Autodesk Inventor part; units mm, degrees
ref_plane "YZ Plane" through (0, 0, 0) normal (1, 0, 0) x (0, 1, 0)
ref_plane "XZ Plane" through (0, 0, 0) normal (0, 1, 0) x (-1, 0, 0)
ref_plane "XY Plane" through (0, 0, 0) normal (0, 0, 1) x (1, 0, 0)
sketch "Sketch1" plane through (0, 0, 0) normal (0, 0, 1) x (1, 0, 0)
  line L0 (45, 15) -> (-5, 15)
  line L1 (-1, 8) -> (-1, 0)
  line L2 (1, 0) -> (1, 8)
  arc A0 (1, 8) -> (-1, 8) centre (0, 8) ccw
  arc A1 (17, 8) -> (15, 8) centre (16, 8) ccw
  line L3 (15, 8) -> (15, 0)
  line L4 (17, 0) -> (17, 8)
  line L5 (2.5, 0) -> (2.5, 0)
  line L6 (22.48, 0) -> (22.48, 0)
  line L7 (-5, 15) -> (-5, 0)
  line L8 (-5, 0) -> (-1, 0)
  line L9 (45, 0) -> (45, 15)
  line L10 (17, 0) -> (45, 0)
  line L11 (1, 0) -> (15, 0)
  point P0 (0, 0)
  point P1 (15, 0)
  dimension "d0" = 50
  dimension "d1" = 15
  dimension "d3" = 2
  dimension "d6" = 0
  dimension "d7" = 16
extrude "Extrusion2" add sketch "Sketch1" along normal blind 3.5
properties part number "C2"
Geometry check sheet. Reference: the model listing, model coordinates, mm. A direction names the side the tool comes from. Round coordinates to 2 decimals unless told otherwise and drop trailing zeros. Write each loop counter-clockwise with the first axis right and the second up, starting at its lowest first coordinate (ties: lowest second). Pieces come first, ordered by that corner, then holes. Notation, with made-up numbers: (14.5, 34) -> (56.5, 34) arc R9 cw to (56.5, 45) -> close; hole circle Ø10 at (25.25, -26). An arc over 180 degrees is marked (long way). One line per item, written item: value. Start each with the question number.
(1) Cross-section at B-B, the plane z = 1.95. Record the cut outline in (x, y), and give its area (3 significant figures).
(2) Draft check along X on faces 3 (the flat face through (-3, 0, 2)), 4 (the cylindrical face through (0, 9, 2)), 5 (the flat face through (45, 7, 2)). Enter one of: +X half, -X half, draft (parallel to the pull), parting line (faces both ways), or undercut.
(3) Scan lines: line 1 (X direction, y = 8, z = 1.8); line 2 (X direction, y = 8.5, z = 2.55). Record each from-to range of solid material in increasing order. Write a range as [from, to].
(4) Cross-section at A-A, the plane y = 6.5. Record the cut outline in (x, z).
(5) Cross-section at C-C, the plane x = 16. Record the cut outline in (y, z).
(6) Access from +Z, -Z, +X, -X, +Y, -Y to the whole of each face (thin tool, end or side, straight path). Record for faces 1 (the flat face through (15, 4, 2)), 2 (the flat face through (-5, 8, 2)).
Answer:
1. outline: (-5, 0) -> (-1, 0) -> (-1, 8) arc R1 cw to (1, 8) -> (1, 0) -> (15, 0) -> (15, 8) arc R1 cw to (17, 8) -> (17, 0) -> (45, 0) -> (45, 15) -> (-5, 15) -> close
1. area: 715 mm²
2. face 3: draft
2. face 4: undercut
2. face 5: +X half
3. line 1: [-5, -1], [1, 15], [17, 45]
3. line 2: [-5, -0.87], [0.87, 15.13], [16.87, 45]
4. outline: (-5, 0) -> (-1, 0) -> (-1, 3.5) -> (-5, 3.5) -> close; (1, 0) -> (15, 0) -> (15, 3.5) -> (1, 3.5) -> close; (17, 0) -> (45, 0) -> (45, 3.5) -> (17, 3.5) -> close
5. outline: (9, 0) -> (15, 0) -> (15, 3.5) -> (9, 3.5) -> close
6. face 1: +Z, -Z, -Y
6. face 2: +Z, -Z, -X, +Y, -Y
